from build123d import *

# Parameters (mm, degrees)
F0_W     = 317.5
F0_H     = 1219.2
F1_DEPTH = 3.4163
F2_W     = 317.5
F2_H     = 3.4163
F3_DEPTH = 110.8837
F4_R     = 7.9375
F5_DEPTH = 3.4173


with BuildPart() as f1:
    # F0 (on Front) → F1 (new body)
    with BuildSketch(Plane.XZ):
        Rectangle(F0_W, F0_H)
    extrude(amount=F1_DEPTH)

    # F2 (on face) → F3 (join)
    with BuildSketch(Plane.XZ.offset(3.4163)):
        with Locations((0, -607.89185)):
            Rectangle(F2_W, F2_H)
    extrude(amount=F3_DEPTH)

    # F4 (on face) → F5 (cut, through all)
    with BuildSketch(Plane.XY.offset(-606.1837)):
        with Locations((-125.4125, -58.85815)):
            Circle(F4_R)
        with Locations((0, -58.85815)):
            Circle(F4_R)
        with Locations((125.4125, -58.85815)):
            Circle(F4_R)
    extrude(amount=-F5_DEPTH, mode=Mode.SUBTRACT)


solid = f1.part
The model under review builds one solid part; all positions refer to its coordinate system, in mm. A direction names the side the tool comes from. Round coordinates to 2 decimals unless told otherwise and drop trailing zeros. Write each loop counter-clockwise with the first axis right and the second up, starting at its lowest first coordinate (ties: lowest second). Pieces come first, ordered by that corner, then holes. Notation, with made-up numbers: M 85.25,79 L 116.25,79 A18 cw 116.25,90 Z; hole C 16.25,56.5 d9. An arc over 180 degrees is marked long. Answer as CSV lines item,"result". Start each with the question number.
Q1. Consider section C-C, the plane y = -78. Give the boundary of the cut face in (x, z).
Q2. Wall thickness on line 1 along Z through (x, y) = (-34, -98); line 2 along Y through (x, z) = (-119, -418.5): over which ranges is each line inside the solid? List them lowest first.
Q3. Clearance check with a flat-ended pin moving along its axis: P1, Ø12, axis at x = 25.5, z = -414, coming from the -Y side. State where the tip first meets the part, or that it passes through.
Q4. Consider section A-A, the plane x = 65. Give the boundary of the cut face in (y, z).
Q5. Consider section B-B, the plane z = 198. Give the boundary of the cut face in (x, y), then the cut area to 3 significant figures.
Q6. Tool access review of faces 1 (the face through (-2, 0, 9)), 2 (the face through (-2, -46, -606.184)): name each direction out of +Z, -Z, +X, -X, +Y, -Y from which nothing blocks a thin tool from reaching the whole face with its end or side.
Result set:
1,outline,"M -158.75,-609.6 L 158.75,-609.6 L 158.75,-606.18 L -158.75,-606.18 Z"
2,line 1,"z = -609.6 to -606.18"
2,line 2,"y = -3.42 to 0"
3,P1,"stops at y = -3.42"
4,outline,"M -114.3,-609.6 L 0,-609.6 L 0,609.6 L -3.42,609.6 L -3.42,-606.18 L -114.3,-606.18 Z"
5,outline,"M -158.75,-3.42 L 158.75,-3.42 L 158.75,0 L -158.75,0 Z"
5,area,"1,080 mm²"
6,face 1,"+Z, -Z, +X, -X, +Y"
6,face 2,"+Z, +X, -X, -Y"
